Autodesk Inventor part; units mm, degrees
ref_plane "YZ Plane" through (0, 0, 0) normal (1, 0, 0) x (0, 1, 0)
ref_plane "XZ Plane" through (0, 0, 0) normal (0, 1, 0) x (-1, 0, 0)
ref_plane "XY Plane" through (0, 0, 0) normal (0, 0, 1) x (1, 0, 0)
sketch "Sketch1" plane through (0, 0, 0) normal (1, 0, 0) x (0, 1, 0)
  line L0 (35.3248, 20.4047) -> (35.3248, -21.0933)
  line L1 (29.1498, -27.2683) -> (-15.4752, -27.2683)
  line L2 (-15.4752, -27.2683) -> (-15.4752, -14.5683)
  line L3 (-15.4752, -14.5683) -> (-22.144, -14.5683)
  line L4 (-27.319, -8.7583) -> (-27.319, 8.0697)
  line L5 (-22.144, 13.8797) -> (-15.4752, 13.8797)
  line L6 (-15.4752, 13.8797) -> (-15.4752, 26.5797)
  line L7 (-15.4752, 26.5797) -> (29.1498, 26.5797)
  circle A0 centre (32.1498, 23.4047) radius 1.524
  circle A1 centre (32.1498, -24.0933) radius 1.524
  circle A2 centre (-24.144, -10.7583) radius 1.524
  circle A3 centre (-24.144, 10.0697) radius 1.524
  arc A4 (32.1498, -21.0933) -> (29.1498, -24.0933) centre (32.1498, -24.0933) ccw
  line L8 (29.1498, -24.0933) -> (29.1498, -27.2683)
  line L9 (32.1498, -21.0933) -> (35.3248, -21.0933)
  line L10 (38.3248, -21.0933) -> (38.3248, -27.2683)
  line L11 (38.3248, -27.2683) -> (38.3248, -30.2683)
  line L12 (38.3248, -30.2683) -> (-15.4752, -30.2683)
  line L13 (-15.4752, -30.2683) -> (-18.4752, -30.2683)
  line L14 (-18.4752, -30.2683) -> (-18.4752, -17.8683)
  line L15 (-18.4752, -17.8683) -> (-27.319, -17.8683)
  line L16 (-27.319, -17.8683) -> (-30.319, -17.8683)
  line L17 (-30.319, -17.8683) -> (-30.319, 13.8797)
  line L18 (-30.319, 13.8797) -> (-30.319, 16.8797)
  line L19 (-30.319, 16.8797) -> (-18.4752, 16.8797)
  line L20 (-18.4752, 16.8797) -> (-18.4752, 26.5797)
  line L21 (-18.4752, 26.5797) -> (-18.4752, 29.5797)
  line L22 (-18.4752, 29.5797) -> (35.3248, 29.5797)
  line L23 (35.3248, 29.5797) -> (38.3248, 29.5797)
  line L24 (38.3248, 29.5797) -> (38.3248, -21.0933)
  line L25 (32.1498, 20.4047) -> (38.3248, 20.4047)
  line L26 (29.1498, 23.4047) -> (29.1498, 29.5797)
  arc A5 (29.1498, 23.4047) -> (32.1498, 20.4047) centre (32.1498, 23.4047) ccw
  line L27 (-24.144, 8.0697) -> (-30.319, 8.0697)
  line L28 (-22.144, 10.0697) -> (-22.144, 16.8797)
  arc A6 (-24.144, 8.0697) -> (-22.144, 10.0697) centre (-24.144, 10.0697) ccw
  line L29 (-24.144, -10.7583) -> (-22.144, -10.7583) construction
  line L30 (-24.144, -8.7583) -> (-30.319, -8.7583)
  line L31 (-22.144, -10.7583) -> (-22.144, -17.8683)
  arc A7 (-22.144, -10.7583) -> (-24.144, -8.7583) centre (-24.144, -10.7583) ccw
  line L32 (35.3248, -21.0933) -> (38.3248, -21.0933)
  line L33 (29.1498, -27.2683) -> (29.1498, -30.2683)
  point P0 (0, 0)
  point P1 (0, 0)
extrude "Extrusion1" add sketch "Sketch1" along normal blind 3 contours L25 L24 L32 L0 | L25 A5 L26 L22 L23 L24 | L32 L10 L11 L12 L33 L8 A4 L9 | L7 L6 L5 L28 L19 L20 L21 L22 L26 | L33 L12 L13 L14 L15 L31 L3 L2 L1 | L28 A6 L27 L17 L18 L19 | L31 L15 L16 L17 L30 A7 | L4 L30 L17 L27
properties part number "pixy mount"
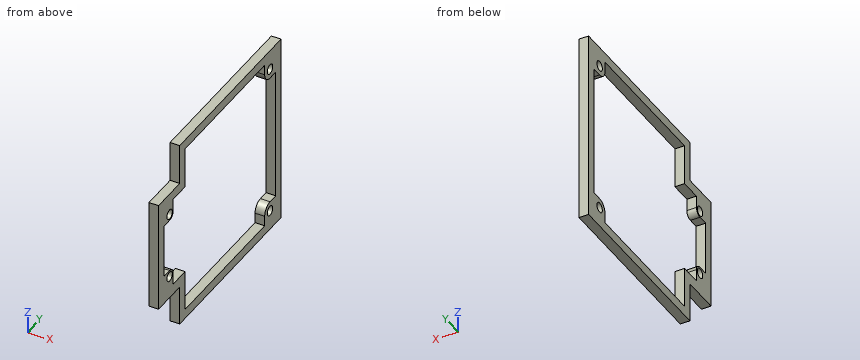
Geometry: final body of the model. Coordinates: model frame, mm. Round coordinates to 2 decimals unless told otherwise and drop trailing zeros. Order: outer loops, then holes, each group sorted by start corner. A loop starts at its lowest first (then second) coordinate and runs counter-clockwise, first axis right, second up. Notation, with made-up numbers: (85, -17) - (122, -17) arc R11 cw to (122, 1) - close; hole circle Ø7 at (62, 89.25). An arc over 180 degrees is marked (long way). Write each question's results on one line, items separated by ' | '.
Item 1: Section C-C, the plane x = 1.85. State how many separate pieces and enclosed holes the cut face has, and give its area (3 significant figures).
Completed:
separate pieces: 1 | enclosed holes: 5 | area: 840 mm^2
Item 2: Section B-B, the plane y = -6.5. Return the cut outline in (x, z), and give its area (3 significant figures).
Completed:
outline: (0, -30.27) - (3, -30.27) - (3, -27.27) - (0, -27.27) - close; (0, 26.58) - (3, 26.58) - (3, 29.58) - (0, 29.58) - close | area: 18.0 mm^2
Item 3: Material intervals for line 1 along Y through (x, z) = (2.3, -24); line 2 along Y through (x, z) = (0.7, 12); line 3 along Z through (x, y) = (0.8, 1), sorted ascending. Write a range as [from, to].
Completed:
line 1: [-18.48, -15.48], [29.15, 30.63], [33.67, 38.32] | line 2: [-30.32, -22.14], [35.32, 38.32] | line 3: [-30.27, -27.27], [26.58, 29.58]
Item 4: Section A-A, the plane z = -16. Return the cut outline in (x, y), and give its area (3 significant figures).
Completed:
outline: (0, -30.32) - (3, -30.32) - (3, -15.48) - (0, -15.48) - close; (0, 35.32) - (3, 35.32) - (3, 38.32) - (0, 38.32) - close | area: 53.5 mm^2
Item 5: First-contact query: pin 1 Ø0.9 at (x, y) = (2, -26) entering from -Z; pin 2 Ø1.5 at (x, y) = (2, -26) entering from +Z; pin 3 Ø0.9 at (x, z) = (1, 26) entering from -Y. Flat tips, straight axial feed; report the tip coordinate or a pass-through.
Completed:
pin 1: z = -17.87 | pin 2: z = 16.88 | pin 3: y = -18.48
